Read the model definition and answer for the solid it produces. Units are mm, in the model's axes. Round coordinates to 2 decimals unless told otherwise and drop trailing zeros. Write each loop counter-clockwise with the first axis right and the second up, starting at its lowest first coordinate (ties: lowest second). Pieces come first, ordered by that corner, then holes. Notation, with made-up numbers: (21, 78) - (48, 78) arc R30 ccw to (48, 100) - close; hole circle Ø3 at (28, -13.5). An arc over 180 degrees is marked (long way). Use one line per item in the form item = value. Start each with the question number.
1) Consider line 1 along X through (y, z) = (10.75, 0); line 2 along X through (y, z) = (13.25, 0.25); line 3 along Z through (x, y) = (0.9, 7). Determine where each line is inside the solid, lowest interval first. Write a range as from..to.
2) For a pull along Z with two mould halves and no side action, classify faces 1 (the face through (-0.97, 7.6, -1.27)), 2 (the face through (2, 15, 0)), 3 (the face through (0, 7, 2.3)) as released by +Z, released by -Z, zero draft, split by the parting line, or undercut.
3) The part is cut by section A-A, the plane z = 0. Give the vertices of the cut face in (x, y), plus the area to 3 significant figures.
4) The part is cut by section D-D, the plane x = 1.95. Give the vertices of the cut face in (y, z), plus the area to 3 significant figures.
5) The part is cut by section C-C, the plane y = 2.25. Give the vertices of the cut face in (x, z).
6) The part is cut by section B-B, the plane x = 0. Give the vertices of the cut face in (y, z).
from build123d import *

# Parameters (mm, degrees)
BOSS_EXTRUDE1_DEPTH = 15
SKETCH2_R           = 1.6
CUT_EXTRUDE1_DEPTH  = 16.405951231
FILLET1_R           = 0.5
CHAMFER1_SIZE       = 0.2


with BuildPart() as part:
    # Sketch1 → Boss-Extrude1 (new body)
    with BuildSketch(Plane(origin=(0, 0, 0), x_dir=(1, 0, 0), z_dir=(0, 1, 0))):
        Polygon((1.327905619, -2.3), (2.655811238, 0), (1.327905619, 2.3), (-1.327905619, 2.3), (-2.655811238, 0), (-1.327905619, -2.3), align=None)
    extrude(amount=BOSS_EXTRUDE1_DEPTH)

    # Sketch2 → Cut-Extrude1 (cut, through all)
    with BuildSketch(Plane(origin=(0, 15, 0), x_dir=(1, 0, 0), z_dir=(0, 1, 0))):
        with Locations(Location((0, 0, 0), (0, 0, 270))):
            Circle(SKETCH2_R)
    extrude(amount=-CUT_EXTRUDE1_DEPTH, mode=Mode.SUBTRACT)

    # Fillet1
    fillet1_edges = [part.edges().sort_by_distance(p)[0] for p in [
        (-1.327905619, 7.5, 2.3),
        (-2.655811238, 7.5, 0),
        (-1.327905619, 7.5, -2.3),
        (1.327905619, 7.5, -2.3),
        (2.655811238, 7.5, 0),
        (1.327905619, 7.5, 2.3),
    ]]
    fillet(fillet1_edges, radius=FILLET1_R)

    # Chamfer1
    chamfer1_edges = [part.edges().sort_by_distance(p)[0] for p in [
        (0, 0, 2.3),
        (0, 15, 2.3),
        (-1.991858429, 0, 1.15),
        (-1.991858429, 0, -1.15),
        (0, 0, -2.3),
        (1.991858429, 0, -1.15),
        (1.991858429, 0, 1.15),
        (1.289230485, 0, 2.233012702),
        (2.578460969, 0, 0),
        (1.289230485, 0, -2.233012702),
        (-1.289230485, 0, -2.233012702),
        (-2.578460969, 0, 0),
        (-1.289230485, 0, 2.233012702),
        (-1.991858429, 15, 1.15),
        (1.991858429, 15, 1.15),
        (1.991858429, 15, -1.15),
        (0, 15, -2.3),
        (-1.991858429, 15, -1.15),
        (1.289230485, 15, 2.233012702),
        (2.578460969, 15, 0),
        (1.289230485, 15, -2.233012702),
        (-1.289230485, 15, -2.233012702),
        (-2.578460969, 15, 0),
        (-1.289230485, 15, 2.233012702),
    ]]
    chamfer(chamfer1_edges, length=CHAMFER1_SIZE)


solid = part.part
Geometry results:
q1.line_1 = -2.58..-1.6, 1.6..2.58
q1.line_2 = -2.51..-1.58, 1.58..2.51
q1.line_3 = -2.3..-1.32, 1.32..2.3
q2.face_1 = undercut
q2.face_2 = zero draft
q2.face_3 = released by +Z
q3.outline = (-2.58, 0.2) - (-2.38, 0) - (-1.6, 0) - (-1.6, 15) - (-2.38, 15) - (-2.58, 14.8) - close; (1.6, 0) - (2.38, 0) - (2.58, 0.2) - (2.58, 14.8) - (2.38, 15) - (1.6, 15) - close
q3.area = 29.3 mm2
q4.outline = (0, -0.82) - (0.2, -1.22) - (14.8, -1.22) - (15, -0.82) - (15, 0.82) - (14.8, 1.22) - (0.2, 1.22) - (0, 0.82) - close
q4.area = 36.5 mm2
q5.outline = (-2.51, -0.25) - (-1.47, -2.05) arc R0.5 ccw to (-1.04, -2.3) - (1.04, -2.3) arc R0.5 ccw to (1.47, -2.05) - (2.51, -0.25) arc R0.5 ccw to (2.51, 0.25) - (1.47, 2.05) arc R0.5 ccw to (1.04, 2.3) - (-1.04, 2.3) arc R0.5 ccw to (-1.47, 2.05) - (-2.51, 0.25) arc R0.5 ccw to start; hole circle Ø3.2 at (0, 0)
q6.outline = (0, -2.1) - (0.2, -2.3) - (14.8, -2.3) - (15, -2.1) - (15, -1.6) - (0, -1.6) - close; (0, 1.6) - (15, 1.6) - (15, 2.1) - (14.8, 2.3) - (0.2, 2.3) - (0, 2.1) - close
